Part model, mm, in its own coordinate system. Round coordinates to 2 decimals unless told otherwise and drop trailing zeros. Write each loop counter-clockwise with the first axis right and the second up, starting at its lowest first coordinate (ties: lowest second). Pieces come first, ordered by that corner, then holes.
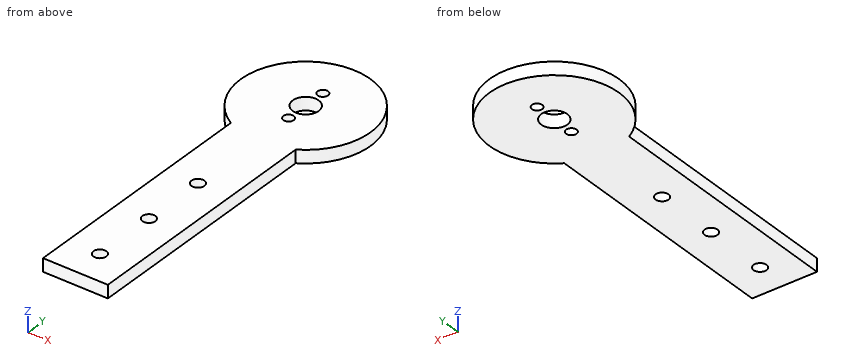
Autodesk Inventor part; units mm, degrees
ref_plane "YZ Plane" through (0, 0, 0) normal (1, 0, 0) x (0, 1, 0)
ref_plane "XZ Plane" through (0, 0, 0) normal (0, 1, 0) x (-1, 0, 0)
ref_plane "XY Plane" through (0, 0, 0) normal (0, 0, 1) x (1, 0, 0)
sketch "スケッチ1" plane through (0, 0, 0) normal (0, 0, 1) x (1, 0, 0)
  circle A0 centre (0, 0) radius 10
  circle A1 centre (0, 0) radius 2
  line L0 (0, -2) -> (0, -47)
  line L1 (10, 0) -> (10, -47)
  line L2 (10, -47) -> (-10, -47)
  line L3 (-10, -47) -> (-10, 0)
  circle A2 centre (0, -32) radius 1
  circle A3 centre (0, -42) radius 1
  circle A4 centre (0, -22) radius 1
  dimension "d1" = 4
  dimension "d0" = 20
  dimension "d2" = 45
  dimension "d9" = 2
  dimension "d10" = 2
  dimension "d11" = 2
extrude "押し出し1" add sketch "スケッチ1" along normal blind 2
sketch "スケッチ2" plane through (0, 0, 2) normal (0, 0, 1) x (1, 0, 0)
  circle A0 centre (0, -32) radius 1
  circle A1 centre (0, -22) radius 1
  circle A2 centre (0, -42) radius 1
  point P0 (0, 0)
  dimension "d12" = 2
  dimension "d13" = 2
  dimension "d14" = 2
extrude "押し出し2" cut sketch "スケッチ2" against normal blind 10
sketch "スケッチ3" plane through (0, 0, 0) normal (0, 0, -1) x (-1, 0, 0)
  line L0 (10, -47) -> (-10, -47)
  line L1 (10, -47) -> (5, -47)
  circle A0 centre (0, 0) radius 10
  line L2 (5, -47) -> (5, -8.660254)
  line L3 (10, 0) -> (10, -47)
  line L4 (10, -47) -> (10, 0)
  line L5 (-10, -47) -> (-10, 0)
  line L6 (-10, 0) -> (-10, -47)
  line L7 (-10, -47) -> (-5, -47)
  line L8 (-5, -47) -> (-5, -8.660254)
  dimension "d17" = 5
  dimension "d18" = 5
sketch "スケッチ3 outline for 押し出し3" plane through (0, 0, 0) normal (0, 0, -1) x (-1, 0, 0)
  line L0 (-5, -47) -> (-5, -8.660254)
  line L1 (-10, -47) -> (-5, -47)
  line L2 (-10, 0) -> (-10, -47)
  arc A0 (-5, -8.660254) -> (-10, 0) centre (0, 0) cw
  line L3 (10, -47) -> (10, 0)
  line L4 (5, -47) -> (10, -47)
  line L5 (5, -8.660254) -> (5, -47)
  arc A1 (10, 0) -> (5, -8.660254) centre (0, 0) cw
extrude "押し出し3" cut sketch "スケッチ3 outline for 押し出し3" against normal blind 10
sketch "スケッチ5" plane through (0, 0, 2) normal (0, 0, 1) x (1, 0, 0)
  circle A0 centre (0, 0) radius 3.5
  circle A1 centre (0, 3.5) radius 0.8
  circle A2 centre (0, -3.5) radius 0.8
  dimension "d31" = 7
  dimension "d32" = 1.6
  dimension "d33" = 1.6
extrude "押し出し5" cut sketch "スケッチ5" against normal blind 10 contours A1 A0 | A0 A1 | A2 A0 | A0 A2
thread "ねじ3"
thread "ねじ4"
properties part number "cutter_board"
Q1. Drop flat-ended pins along their axis: pin 1 (1.6 mm diameter, centred on x = 0, y = -22, fed in from -Z) (3 decimals); pin 2 (1 mm diameter, centred on y = -25.5, z = 1, fed in from -X); pin 3 (1 mm diameter, centred on x = -5.5, z = 0.5, fed in from +Y). Give the stop position or say it passes through.
Values follow:
pin 1: passes through
pin 2: stops at x = -5
pin 3: stops at y = 8.66
Q2. Cut at D-D on y = 0. Write the cut outline in (x, z).
Values follow:
outline: (-10, 0) - (-2, 0) - (-2, 2) - (-10, 2) - close; (2, 0) - (10, 0) - (10, 2) - (2, 2) - close
Q3. Cut at C-C on z = 0.6. Write the cut outline in (x, y), plus the area to 3 significant figures.
Values follow:
outline: (-5, -47) - (5, -47) - (5, -8.66) arc R10 ccw (long way) to (-5, -8.66) - close; hole circle Ø4 at (0, 0); hole circle Ø2 at (0, -42); hole circle Ø2 at (0, -32); hole circle Ø2 at (0, -22); hole circle Ø1.6 at (0, -3.5); hole circle Ø1.6 at (0, 3.5)
area: 662 mm2
Q4. Cut at A-A on x = 0. Write the cut outline in (y, z), plus the area to 3 significant figures.
Values follow:
outline: (-47, 0) - (-43, 0) - (-43, 2) - (-47, 2) - close; (-41, 0) - (-33, 0) - (-33, 2) - (-41, 2) - close; (-31, 0) - (-23, 0) - (-23, 2) - (-31, 2) - close; (-21, 0) - (-4.3, 0) - (-4.3, 2) - (-21, 2) - close; (-2.7, 0) - (-2, 0) - (-2, 2) - (-2.7, 2) - close; (2, 0) - (2.7, 0) - (2.7, 2) - (2, 2) - close; (4.3, 0) - (10, 0) - (10, 2) - (4.3, 2) - close
area: 87.6 mm2
Q5. Cut at B-B on y = -32. Write the cut outline in (x, z).
Values follow:
outline: (-5, 0) - (-1, 0) - (-1, 2) - (-5, 2) - close; (1, 0) - (5, 0) - (5, 2) - (1, 2) - close
Q6. Wall check: L1, parallel to X at y = -19, z = 1.85; L2, parallel to X at y = -3.5, z = 1.2; L3, parallel to Y at x = -6.5, z = 1.8. Give the ranges that are in metal, low to high.
Values follow:
L1: x = -5 to 5
L2: x = -9.37 to -0.8, 0.8 to 9.37
L3: y = -7.6 to 7.6
